from build123d import *

# Parameters (mm, degrees)
F2_R     = 70
F3_DEPTH = 500


with BuildPart() as f1:
    # F0 (on Front) → F1 (revolve)
    with BuildSketch(Plane.XZ):
        with BuildLine():
            Line((70, 440), (0, 440))
            Line((0, 440), (0, 0))
            Line((0, 0), (120, 0))
            Line((120, 0), (120, 30))
            Line((120, 30), (130, 30))
            ThreePointArc((130, 30), (165.355339, 44.644661), (180, 80))
            Line((180, 80), (180, 310))
            ThreePointArc((180, 310), (165.355339, 345.355339), (130, 360))
            Line((130, 360), (90, 360))
            Line((90, 360), (90, 420))
            ThreePointArc((90, 420), (84.142136, 434.142136), (70, 440))
        make_face()
    revolve(axis=Axis((0, 0, 220), (0, 0, -1)))

    # F2 (on face) → F3 (cut)
    with BuildSketch(Plane.XY.offset(440)):
        Circle(F2_R)
    extrude(amount=-F3_DEPTH, mode=Mode.SUBTRACT)


solid = f1.part
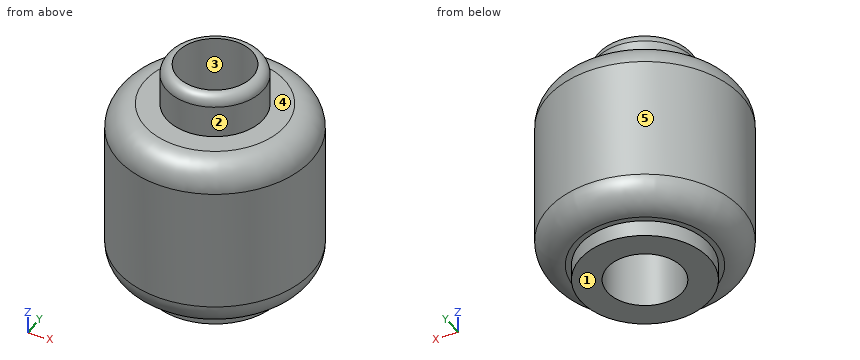
Geometry check sheet. Reference: the model listing, model coordinates, mm. Face numbers are marked on the shaded views. A direction names the side the tool comes from. Give positions to 0.01 mm unless a question says otherwise; leave off trailing zeros. Order: outer loops, then holes, each group sorted by start corner. A loop starts at its lowest first (then second) coordinate and runs counter-clockwise, first axis right, second up. Notation, with made-up numbers: M 13,77 L 32,77 A21 cw 32,81 Z; hole C -5,44.25 d4. An arc over 180 degrees is marked long. Use a Markdown table: item, result.
Item 1: Section check C-C (z = 101.5). Record the cut outline in (x, y), and give its area (3 significant figures).
Answers follow:
| item | result |
|---|---|
| outline | C 0,0 d360; hole C 0,0 d140 |
| area | 86,400 mm2 |
Item 2: Draft check along X on the marked faces 1, 2 and 3. Enter one of: +X half, -X half, draft (parallel to the pull), parting line (faces both ways), or undercut.
Answers follow:
| item | result |
|---|---|
| face 1 | draft |
| face 2 | parting line |
| face 3 | undercut |
Item 3: Tool access check on the marked faces 4 and 5. Record the directions out of +Z, -Z, +X, -X, +Y, -Y that give a thin tool (end or side, any length) a straight path to the whole face; none if there is none.
Answers follow:
| item | result |
|---|---|
| face 4 | +Z |
| face 5 | +Z, -Z |
Item 4: Section check A-A (x = 0). Record the cut outline in (y, z).
Answers follow:
| item | result |
|---|---|
| outline | M -180,80 A50 ccw -130,30 L -120,30 L -120,0 L -70,0 L -70,440 A20 ccw -90,420 L -90,360 L -130,360 A50 ccw -180,310 Z; M 70,0 L 120,0 L 120,30 L 130,30 A50 ccw 180,80 L 180,310 A50 ccw 130,360 L 90,360 L 90,420 A20 ccw 70,440 Z |
Item 5: Material ranges on line 1 along Y through (x, z) = (0, 140.5); line 2 along X through (y, z) = (53, 248.5), recorded low to high.
Answers follow:
| item | result |
|---|---|
| line 1 | y = -180 to -70, 70 to 180 |
| line 2 | x = -172.02 to -45.73, 45.73 to 172.02 |
Item 6: Section check D-D (z = 369.5). Record the cut outline in (x, y), and give its area (3 significant figures).
Answers follow:
| item | result |
|---|---|
| outline | C 0,0 d180; hole C 0,0 d140 |
| area | 10,100 mm2 |
Item 7: Depth check by flat-ended pin: P1, Ø2, axis at x = 98.5, z = 337.5, coming from the +Y side; P2, Ø1, axis at x = -28.5, z = 325.5, coming from the +Y side; P3, Ø3, axis at y = -116.5, z = 321.5, coming from the +X side. Enter the tip coordinate at first touch or a pass-through.
Answers follow:
| item | result |
|---|---|
| P1 | stops at y = 141.76 |
| P2 | stops at y = 175.42 |
| P3 | stops at x = 136.81 |
